```python
from build123d import *

# Parameters (mm, degrees)
BOSS_EXTRUDE1_DEPTH = 2
SCALE1_SCALE        = 2
SKETCH6_R           = 1.5
CUT_EXTRUDE2_DEPTH  = 3
SKETCH10_R          = 1.5
CUT_EXTRUDE4_DEPTH  = 10


with BuildPart() as part:
    # Sketch2 → Boss-Extrude1 (new body)
    with BuildSketch(Plane(origin=(0, 0, 0), x_dir=(1, 0, 0), z_dir=(0, 1, 0))):
        with BuildLine():
            Line((-17.967387551, 9.159795774), (-20.639475337, 7.15016677))
            ThreePointArc((-20.639475337, 7.15016677), (-18.649238809, 4.17439457), (-19.346117765, 0.662896123))
            ThreePointArc((-19.346117765, 0.662896123), (-19.45411943, -1.286546543), (-18.558961711, -3.021678736))
            ThreePointArc((-18.558961711, -3.021678736), (-16.421478173, -5.190969631), (-13.78312899, -6.712078584))
            ThreePointArc((-13.78312899, -6.712078584), (-13.032173848, -6.916004841), (-12.276686285, -7.102440046))
            ThreePointArc((-12.276686285, -7.102440046), (-12.194265553, -8.245293076), (-11.737308023, -9.296052821))
            ThreePointArc((-11.737308023, -9.296052821), (-10.975506649, -9.937799505), (-10.090124565, -10.394175126))
            Line((-10.090124565, -10.394175126), (-7.391598262, -11.698651137))
            Line((-7.391598262, -11.698651137), (7.391598262, -11.698651137))
            Line((7.391598262, -11.698651137), (10.090124565, -10.394175126))
            ThreePointArc((10.090124565, -10.394175126), (10.975506649, -9.937799505), (11.737308023, -9.296052821))
            ThreePointArc((11.737308023, -9.296052821), (12.194265553, -8.245293076), (12.276686285, -7.102440046))
            ThreePointArc((12.276686285, -7.102440046), (13.032173848, -6.916004841), (13.78312899, -6.712078584))
            ThreePointArc((13.78312899, -6.712078584), (16.421478173, -5.190969631), (18.558961711, -3.021678736))
            ThreePointArc((18.558961711, -3.021678736), (19.45411943, -1.286546543), (19.346117765, 0.662896123))
            ThreePointArc((19.346117765, 0.662896123), (18.649238809, 4.17439457), (20.639475337, 7.15016677))
            Line((20.639475337, 7.15016677), (17.967387551, 9.159795774))
            ThreePointArc((17.967387551, 9.159795774), (10.858325227, 7.499674132), (4.169484372, 10.424426945))
            Line((4.169484372, 10.424426945), (2.224138848, 10.424426945))
            Line((2.224138848, 10.424426945), (0.696104526, 13.114793475))
            Line((0.696104526, 13.114793475), (0, 13.358013588))
            Line((0, 13.358013588), (-0.696104526, 13.114793475))
            Line((-0.696104526, 13.114793475), (-2.224138848, 10.424426945))
            Line((-2.224138848, 10.424426945), (-4.169484372, 10.424426945))
            ThreePointArc((-4.169484372, 10.424426945), (-10.858325227, 7.499674132), (-17.967387551, 9.159795774))
        make_face()
    extrude(amount=BOSS_EXTRUDE1_DEPTH)


with BuildPart() as part_1:
    # Scale1: scaled about (0, 1, 0.242383844)
    add(part.part.scale(SCALE1_SCALE).moved(Location((0, -1, -0.242383844))))

    # Sketch6 → Cut-Extrude2 (cut)
    with BuildSketch(Plane(origin=(0, 3, 0), x_dir=(1, 0, 0), z_dir=(0, 1, 0))):
        with Locations(Location((-5.851533015, 16.28357055, 0), (0, 0, 270))):
            Circle(SKETCH6_R)
        with Locations(Location((4.151829214, 16.28357055, 0), (0, 0, 270))):
            Circle(SKETCH6_R)
    extrude(amount=-CUT_EXTRUDE2_DEPTH, mode=Mode.SUBTRACT)

    # Sketch10 → Cut-Extrude4 (cut)
    with BuildSketch(Plane(origin=(0, 3, 0), x_dir=(1, 0, 0), z_dir=(0, 1, 0))):
        with Locations(Location((-0.8498519, -20.895328087, 0), (0, 0, 270))):
            Circle(SKETCH10_R)
    extrude(amount=-CUT_EXTRUDE4_DEPTH, mode=Mode.SUBTRACT)


solid = part_1.part
```
CAD build for the part. Positions are in the model's coordinates, mm. A direction names the side the tool comes from. Coordinates: 2 decimals unless noted, no trailing zeros. Loops run counter-clockwise (first coordinate to the right, second up) from the corner with the lowest first, then second, coordinate; pieces in that order, holes last. Notation, with made-up numbers: (0.5, 4) - (5.5, 4) arc R27 ccw to (5.5, 28) - close; hole circle Ø6 at (15.5, 72.25). An arc over 180 degrees is marked (long way). Use CSV: the item, a comma, the result in double quotes. Start each with the question number.
Q1. Drop flat-ended pins along their axis: P1, Ø1.2, axis at x = -5.5, y = 2, coming from the -Z side; P2, Ø2, axis at x = 23, y = 0, coming from the +Z side; P3, Ø1, axis at y = 1, z = -4.5, coming from the -X side (3 decimals). Give the stop position or say it passes through.
Q2. Cut at C-C, the plane z = -8. List the corners of the cut face in (x, y).
Q3. Two-plate mould, pull along Z, no slides. Class faces 1 (the cylindrical face through (3.577, 1.521, -14.898)), 2 (the cylindrical face through (-22, 1, 19.6)), 3 (the flat face through (2.942, 0.972, -23.744)), 4 (the cylindrical face through (-0.784, 1.028, 19.397)): +Z half, -Z half, draft (parallel to the pull), parting line (faces both ways), or undercut.
Q4. Probe probe 1 along Z at (x, y) = (8, 2.55); probe 2 along X at (y, z) = (0.3, -15); probe 3 along X at (y, z) = (-0.75, 12). List the from-to ranges inside material, lowest first. Write a range as from..to.
Q5. Cut at B-B, the plane x = -11. List the corners of the cut face in (y, z), then the cut area to 3 significant figures.
Q6. 3-axis set-ups, long thin cutter, end or side, ignore diameter. For faces 5 (the cylindrical face through (-6.43, 1.52, -14.9)), 6 (the flat face through (-6, 1, -21.091)), 7 (the cylindrical face through (-32.91, 0.97, 10.09)): which of +Z, -Z, +X, -X, +Y, -Y reach the whole face in a straight line?
Q7. Cut at A-A, the plane y = 2.2. List the corners of the cut face in (x, z), then the cut area to 3 significant figures.
Here are the results:
1,P1,"z = -21.09"
1,P2,"z = 19.6"
1,P3,"x = -37.535"
2,outline,"(-37.2, -1) - (37.2, -1) - (37.2, 3) - (-37.2, 3) - close"
3,face 1,"undercut"
3,face 2,"+Z half"
3,face 3,"-Z half"
3,face 4,"undercut"
4,probe 1,"-21.09..23.15"
4,probe 2,"-40.67..-6.63, -5.08..3.38, 4.93..40.67"
4,probe 3,"-30.02..30.02"
5,outline,"(-1, -19.03) - (3, -19.03) - (3, 23.15) - (-1, 23.15) - close"
5,area,"169 mm2"
6,face 5,"+Y"
6,face 6,"-Z, -X, +Y, -Y"
6,face 7,"+Z, -X, +Y, -Y"
7,outline,"(-41.28, -14.54) - (-35.93, -18.56) arc R23.15 cw to (-8.34, -21.09) - (-4.45, -21.09) - (-1.39, -26.47) - (0, -26.96) - (1.39, -26.47) - (4.45, -21.09) - (8.34, -21.09) arc R23.15 cw to (35.93, -18.56) - (41.28, -14.54) arc R9.35 cw to (38.69, -1.57) arc R7.43 ccw to (37.12, 5.8) arc R22.64 ccw to (27.57, 13.18) arc R67.02 ccw to (24.55, 13.96) arc R6.81 ccw to (23.47, 18.35) arc R8.91 ccw to (20.18, 20.55) - (14.78, 23.15) - (-14.78, 23.15) - (-20.18, 20.55) arc R8.91 ccw to (-23.47, 18.35) arc R6.81 ccw to (-24.55, 13.96) arc R67.02 ccw to (-27.57, 13.18) arc R22.64 ccw to (-37.12, 5.8) arc R7.43 ccw to (-38.69, -1.57) arc R9.35 cw to start; hole circle Ø3 at (-5.85, -16.28); hole circle Ø3 at (-0.85, 20.9); hole circle Ø3 at (4.15, -16.28)"
7,area,"2,750 mm2"
